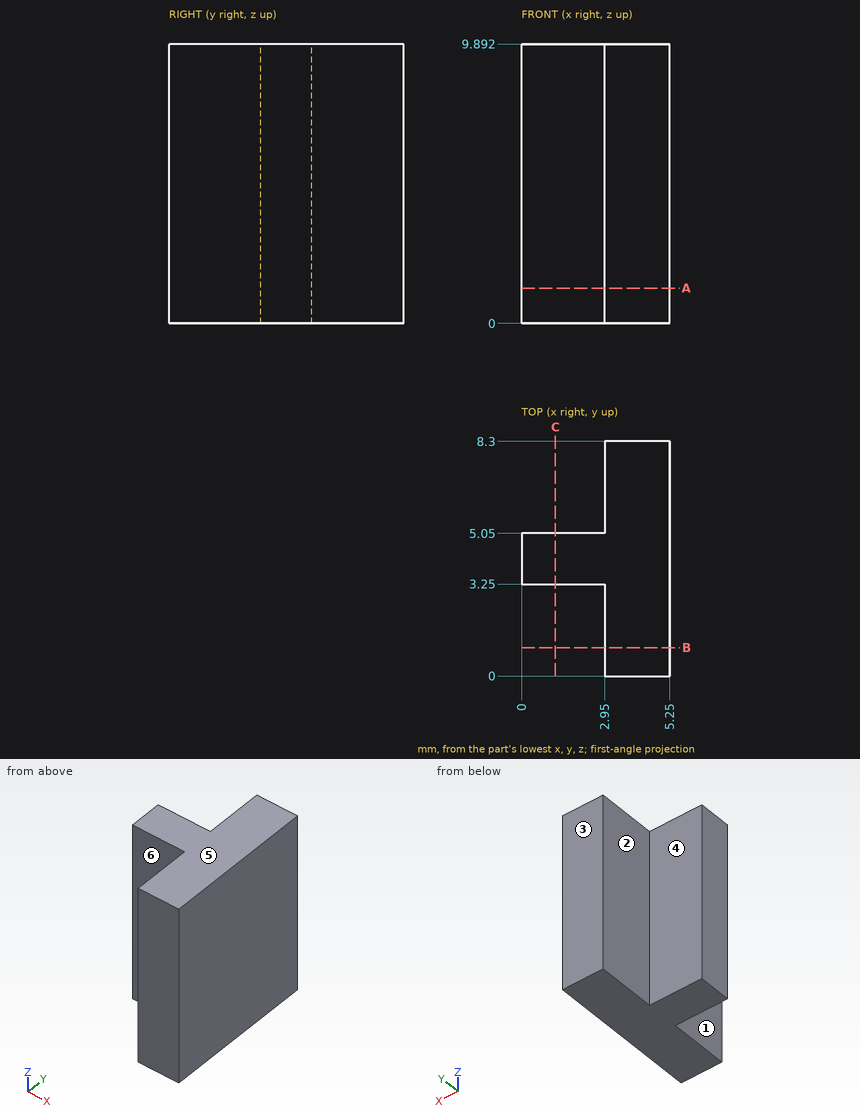
Source: three-view drawing plus pictorial views. Frame: mm from the lowest corner of the part. A direction names the side the tool comes from. Round coordinates to 2 decimals unless told otherwise and drop trailing zeros. Loops run counter-clockwise (first coordinate to the right, second up) from the corner with the lowest first, then second, coordinate; pieces in that order, holes last.
Q1. Section C-C, the plane x = 1.2. Return loops of the section in (y, z), plus the area to 3 significant figures.
Q2. Access query for the marked faces 1, 2 and 3. Directions: +Z, -Z, +X, -X, +Y, -Y. A direction counts if a zero-diameter tool reaches every point of the face in a straight line with its end or side. Return the directions, or none.
Q3. First-contact query: P1, Ø0.9, axis at x = 1.5, z = 3.5, coming from the +Y side; P2, Ø1.6, axis at y = 1.5, z = 5, coming from the -X side; P3, Ø1.5, axis at x = 1, z = 6.5, coming from the -Y side. Flat tips, straight axial feed; report the tip coordinate or a pass-through.
Q4. Mould query, pull axis Y, two halves, no side actions, for the marked faces 4, 5 and 6. Classes: pulls with the +Y half, pulls with the -Y half, needs draft (parallel to the pull), parting line crosses it, or undercut.
Q5. Section B-B, the plane y = 1. Return loops of the section in (x, z), plus the area to 3 significant figures.
Q6. Ray query, line 1 (X direction, y = 5.75, z = 4); line 2 (Y direction, x = 0.7, z = 7.75). Return the intervals inside material, ascending.
Q7. Section A-A, the plane z = 1.25. Return loops of the section in (x, y).
Solutions:
1. outline: (3.25, 0) - (5.05, 0) - (5.05, 9.89) - (3.25, 9.89) - close
1. area: 17.8 mm2
2. face 1: +Z, -Z, -X, -Y
2. face 2: +Z, -Z, -X, +Y
2. face 3: +Z, -Z, +X, -X, +Y
3. P1: stops at y = 5.05
3. P2: stops at x = 2.95
3. P3: stops at y = 3.25
4. face 4: pulls with the +Y half
4. face 5: needs draft
4. face 6: pulls with the -Y half
5. outline: (2.95, 0) - (5.25, 0) - (5.25, 9.89) - (2.95, 9.89) - close
5. area: 22.8 mm2
6. line 1: x = 2.95 to 5.25
6. line 2: y = 3.25 to 5.05
7. outline: (0, 3.25) - (2.95, 3.25) - (2.95, 0) - (5.25, 0) - (5.25, 8.3) - (2.95, 8.3) - (2.95, 5.05) - (0, 5.05) - close
